Here's the drawing with two shaded views (mm, measured from the low corner). I have some questions. Coordinates: 2 decimals unless noted, no trailing zeros. Write each loop counter-clockwise with the first axis right and the second up, starting at its lowest first coordinate (ties: lowest second). Pieces come first, ordered by that corner, then holes. Notation, with made-up numbers: (-16, 49) - (21, 49) arc R30 ccw to (21, 72) - close; hole circle Ø1 at (20, -21.75). An arc over 180 degrees is marked (long way). Answer in a Markdown table with one row per item. Add a question column.
Item 1: I'm going to push a flat-ended pin straight in: pin 1 (1.6 mm diameter, centred on x = 30, z = 2.5, fed in from +Y). Where does the tip first touch, or does it pass through?
Item 2: If I drill on probe 1 along Z at (x, y) = (30, 5); probe 2 along X at (y, z) = (5.25, 2.5); probe 3 along X at (y, z) = (4.25, 2.1), over which ranges is the centre line in solid material (lowest first)? Write a range as from..to.
Item 3: Imagine slicing it at B-B (x = 30). Please give me the cut outline in (y, z).
Item 4: Imagine slicing it at A-A (z = 2.5). Please give me the cut outline in (x, y).
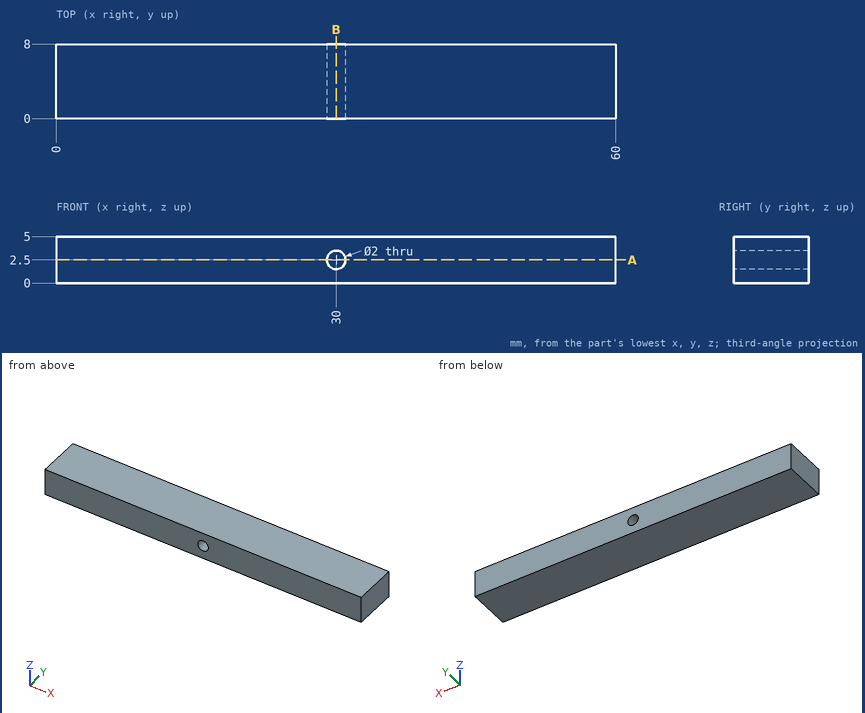
Here are the results:
| question | item | result |
|---|---|---|
| 1 | pin 1 | passes through |
| 2 | probe 1 | z = 0..1.5, 3.5..5 |
| 2 | probe 2 | x = 0..29, 31..60 |
| 2 | probe 3 | x = 0..29.08, 30.92..60 |
| 3 | outline | (0, 0) - (8, 0) - (8, 1.5) - (0, 1.5) - close; (0, 3.5) - (8, 3.5) - (8, 5) - (0, 5) - close |
| 4 | outline | (0, 0) - (29, 0) - (29, 8) - (0, 8) - close; (31, 0) - (60, 0) - (60, 8) - (31, 8) - close |
